from build123d import *

# Parameters (mm, degrees)
BOSS_EXTRUDE1_DEPTH      = 25
BOSS_EXTRUDE1_DEPTH_BACK = 25
SKETCH3_R                = 11.05
SKETCH3_R_2              = 1.75
CUT_EXTRUDE1_DEPTH       = 55
CUT_EXTRUDE2_DEPTH       = 51
CHAMFER1_SIZE            = 5
FILLET1_R                = 2
FILLET2_R                = 3.5
BOSS_EXTRUDE2_DEPTH      = 2.5
SKETCH6_R                = 3.175
BOSS_EXTRUDE3_DEPTH      = 15


with BuildPart() as part:
    # Sketch1 → Boss-Extrude1 (new body, two sides)
    with BuildSketch(Plane(origin=(0, 0, 0), x_dir=(0, 0, -1), z_dir=(1, 0, 0))) as boss_extrude1_sk:
        Polygon((-50, 0), (-50, -2.8), (-2.8, -2.8), (-2.8, -54), (0, -54), (0, 0), align=None)
    extrude(amount=BOSS_EXTRUDE1_DEPTH)
    extrude(boss_extrude1_sk.sketch, amount=-BOSS_EXTRUDE1_DEPTH_BACK)

    # Sketch3 → Cut-Extrude1 (cut, through all)
    with BuildSketch(Plane(origin=(0, 0, 0), x_dir=(1, 0, 0), z_dir=(0, 1, 0))):
        with Locations((0, -29)):
            Circle(SKETCH3_R)
        with Locations((-15.5, -13.5)):
            Circle(SKETCH3_R_2)
        with Locations((15.5, -13.5)):
            Circle(SKETCH3_R_2)
        with Locations((15.5, -44.5)):
            Circle(SKETCH3_R_2)
        with Locations((-15.5, -44.5)):
            Circle(SKETCH3_R_2)
    extrude(amount=-CUT_EXTRUDE1_DEPTH, mode=Mode.SUBTRACT)

    # Sketch4 → Cut-Extrude2 (cut, through all)
    with BuildSketch(Plane(origin=(0, 0, 0), x_dir=(-1, 0, 0), z_dir=(0, 0, -1))):
        with BuildLine():
            Line((-17.1, -43), (-17.1, -13))
            ThreePointArc((-17.1, -13), (-15, -10.9), (-12.9, -13))
            Line((-12.9, -13), (-12.9, -43))
            ThreePointArc((-12.9, -43), (-15, -45.1), (-17.1, -43))
        make_face()
        with BuildLine():
            Line((12.9, -43), (12.9, -13))
            ThreePointArc((12.9, -13), (15, -10.9), (17.1, -13))
            Line((17.1, -13), (17.1, -43))
            ThreePointArc((17.1, -43), (15, -45.1), (12.9, -43))
        make_face()
    extrude(amount=-CUT_EXTRUDE2_DEPTH, mode=Mode.SUBTRACT)

    # Chamfer1
    chamfer1_edges = [part.edges().sort_by_distance(p)[0] for p in [
        (25, -1.4, 50),
        (25, -54, 1.4),
        (-25, -54, 1.4),
        (-25, -1.4, 50),
    ]]
    chamfer(chamfer1_edges, length=CHAMFER1_SIZE)

    # Fillet1
    fillet1_edges = [part.edges().sort_by_distance(p)[0] for p in [
        (0, -2.8, 2.8),
    ]]
    fillet(fillet1_edges, radius=FILLET1_R)

    # Fillet2
    fillet2_edges = [part.edges().sort_by_distance(p)[0] for p in [
        (0, 0, 0),
    ]]
    fillet(fillet2_edges, radius=FILLET2_R)

    # Sketch5 → Boss-Extrude2 (add)
    with BuildSketch(Plane.ZY.offset(25)):
        Polygon((2.8, -5.3), (5.3, -2.8), (22, -2.8), (2.8, -16), align=None)
    boss_extrude2 = extrude(amount=-BOSS_EXTRUDE2_DEPTH)

    # Mirror1: Boss-Extrude2 across plane
    add(boss_extrude2.mirror(Plane(origin=(0, 0, 0), x_dir=(0, 0, 1), z_dir=(1, 0, 0))))

    # Sketch6 → Boss-Extrude3 (add)
    with BuildSketch(Plane.XY.offset(2.8)):
        with Locations((0, -29)):
            Circle(SKETCH6_R)
    extrude(amount=-BOSS_EXTRUDE3_DEPTH)


solid = part.part
Geometry: final body of the model. Coordinates: model frame, mm. A direction names the side the tool comes from. Coordinates: 2 decimals unless noted, no trailing zeros. Loops run counter-clockwise (first coordinate to the right, second up) from the corner with the lowest first, then second, coordinate; pieces in that order, holes last. Notation, with made-up numbers: (-19.75, 31) - (18.25, 31) arc R35 ccw to (18.25, 66) - close; hole circle Ø2 at (-29.75, 23). An arc over 180 degrees is marked (long way). Put each result on its own line as item: value. Start each with the question number.
Q1. Cut plane B-B, the plane x = 7. Return loops of the section in (y, z).
Q2. Pin query (flat end, axial travel): pin 1 Ø4 at (x, y) = (2, -45.5) entering from +Z; pin 2 Ø6 at (x, y) = (6.5, -27.5) entering from -Z; pin 3 Ø22.5 at (x, z) = (11.5, 27) entering from -Y; pin 4 Ø10 at (y, z) = (-13, 13) entering from +X. Return the tip coordinate at first contact, or that it passes through.
Q3. Pull-direction query (Z, two-part tool) for faces 4 (the cylindrical face through (15.12, -1.38, 46.21)), 5 (the flat face through (-23, -1, 47)), 6 (the flat face through (22.5, -6, 8)); classes: released by +Z, released by -Z, zero draft, split by the parting line, or undercut.
Q4. Set-up query: faces 1 (the flat face through (12.9, -28, 1)), 2 (the cylindrical face through (-0.69, -32.1, -6.01)), 3 (the flat face through (-22.5, -6, 8)). Return all of +Z, -Z, +X, -X, +Y, -Y with unobstructed straight access to the full face (end or side cutting, diameter ignored); none if empty.
Q5. Cut plane D-D, the plane x = -15. Return loops of the section in (y, z).
Q6. Line query: line 1 (X direction, y = -0.95, z = 13.5); line 2 (X direction, y = -2.2, z = 29); line 3 (Z direction, x = 15.5, y = -0.85). Output: solid intervals per line, ascending.
Q7. Cut plane A-A, the plane y = -39. Return loops of the section in (x, z).
Q8. Cut plane C-C, the plane z = 13.5. Return loops of the section in (x, y).
Filled sheet:
1. outline: (-54, 0) - (-3.5, 0) arc R3.5 ccw to (0, 3.5) - (0, 20.45) - (-2.8, 20.45) - (-2.8, 4.8) arc R2 cw to (-4.8, 2.8) - (-54, 2.8) - close; (-2.8, 37.55) - (0, 37.55) - (0, 50) - (-2.8, 50) - close
2. pin 1: z = 2.8
2. pin 2: z = 0
2. pin 3: y = -2.8
2. pin 4: x = 25
3. face 4: undercut
3. face 5: released by +Z
3. face 6: zero draft
4. face 1: +Z, -Z
4. face 2: -Z
4. face 3: +Z, -Y
5. outline: (-54, 0) - (-45.1, 0) - (-45.1, 2.8) - (-54, 2.8) - close; (-10.9, 0) - (-3.5, 0) arc R3.5 ccw to (0, 3.5) - (0, 11.82) - (-2.8, 11.82) - (-2.8, 4.8) arc R2 cw to (-4.8, 2.8) - (-10.9, 2.8) - close; (-2.8, 15.18) - (0, 15.18) - (0, 42.82) - (-2.8, 42.82) - close; (-2.8, 46.18) - (0, 46.18) - (0, 50) - (-2.8, 50) - close
6. line 1: -25 to -17.25, -13.75 to 13.75, 17.25 to 25
6. line 2: -25 to -11.05, 11.05 to 25
6. line 3: 1.21 to 11.75, 15.25 to 42.75, 46.25 to 50
7. outline: (-25, 0) - (-17.1, 0) - (-17.1, 2.8) - (-25, 2.8) - close; (-12.9, 0) - (12.9, 0) - (12.9, 2.8) - (-12.9, 2.8) - close; (17.1, 0) - (25, 0) - (25, 2.8) - (17.1, 2.8) - close
8. outline: (-25, -8.64) - (-22.5, -8.64) - (-22.5, -2.8) - (-17.25, -2.8) - (-17.25, 0) - (-25, 0) - close; (-13.75, -2.8) - (13.75, -2.8) - (13.75, 0) - (-13.75, 0) - close; (17.25, -2.8) - (22.5, -2.8) - (22.5, -8.64) - (25, -8.64) - (25, 0) - (17.25, 0) - close
